```python
from build123d import *

# Parameters (mm, degrees)
SKETCH_1_R               = 75
EXTRUDE_1_DEPTH          = 20
F_4_0MM_1_D              = 4
PATTERN_CIRCULAR_1_COUNT = 4
PATTERN_CIRCULAR_2_COUNT = 6
CUT_EXTRUDE_1_REACH      = 109.935
SKETCH_7_R               = 5
F_4_0MM_2_D              = 4
PATTERN_CIRCULAR_3_COUNT = 2


with BuildPart() as part:
    # 草圖1 → 填料-伸長1 (new body)
    with BuildSketch(Plane.XY):
        Circle(SKETCH_1_R)
    extrude(amount=EXTRUDE_1_DEPTH)

    # Ø4.0mm 定位孔1 (through all)
    with Locations(Plane.XY.offset(20)):
        with Locations((29.69848481, 29.69848481)):
            f_4_0mm_1 = Hole(F_4_0MM_1_D / 2)

    # 環狀複製排列1: Ø4.0mm 定位孔1 ×4 about axis
    pattern_circular_1_axis = Axis((0, 0, 0), (0, 0, 1))
    for i in range(1, PATTERN_CIRCULAR_1_COUNT):
        add(f_4_0mm_1.rotate(pattern_circular_1_axis, i * 360 / PATTERN_CIRCULAR_1_COUNT), mode=Mode.SUBTRACT)

    # 草圖6 → Ø6.0mm 定位孔1 (revolve, cut)
    with BuildSketch(Plane(origin=(0, 75, 10), x_dir=(0, 0, 1), z_dir=(1, 0, 0))):
        Polygon((0, 0), (0, 21.802581857), (3, 20), (3, 0), align=None)
    f_6_0mm_1 = revolve(axis=Axis((0, 81.35, 10), (0, -1, 0)), mode=Mode.SUBTRACT)

    # 環狀複製排列2: Ø6.0mm 定位孔1 ×6 about axis
    pattern_circular_2_axis = Axis((0, 0, -88.99), (0, 0, 1))
    for i in range(1, PATTERN_CIRCULAR_2_COUNT):
        add(f_6_0mm_1.rotate(pattern_circular_2_axis, i * 360 / PATTERN_CIRCULAR_2_COUNT), mode=Mode.SUBTRACT)

    # 草圖7 → 除料-伸長1 (cut, up to next)
    with BuildSketch(Plane.XY.offset(20), mode=Mode.PRIVATE) as cut_extrude_1_sk1:
        Circle(SKETCH_7_R)
    cut_extrude_1_tool1 = extrude(cut_extrude_1_sk1.sketch, amount=-CUT_EXTRUDE_1_REACH, mode=Mode.PRIVATE) & part.part
    add(cut_extrude_1_tool1.solids().sort_by_distance((0, 0, 20))[0], mode=Mode.SUBTRACT)

    # Ø4.0mm 定位孔2 (through all)
    with Locations(Plane.XY.offset(20)):
        with Locations((-42, 0)):
            f_4_0mm_2 = Hole(F_4_0MM_2_D / 2)

    # 環狀複製排列3: Ø4.0mm 定位孔2 ×2 about axis
    pattern_circular_3_axis = Axis((0, 0, 0), (0, 0, 1))
    for i in range(1, PATTERN_CIRCULAR_3_COUNT):
        add(f_4_0mm_2.rotate(pattern_circular_3_axis, i * 360 / PATTERN_CIRCULAR_3_COUNT), mode=Mode.SUBTRACT)


solid = part.part
```
The listing builds one solid part. Answer for the finished solid, in the listing's coordinates (mm). A direction names the side the tool comes from. Give positions to 0.01 mm unless a question says otherwise; leave off trailing zeros. Order: outer loops, then holes, each group sorted by start corner. A loop starts at its lowest first (then second) coordinate and runs counter-clockwise, first axis right, second up.
Item 1: The part is cut by section C-C, the plane z = 15. Give the vertices of the cut face in (x, y).
From the geometry:
outline: circle Ø150 at (0, 0); hole circle Ø4 at (-42, 0); hole circle Ø4 at (-29.7, -29.7); hole circle Ø4 at (-29.7, 29.7); hole circle Ø10 at (0, 0); hole circle Ø4 at (29.7, -29.7); hole circle Ø4 at (29.7, 29.7); hole circle Ø4 at (42, 0)
Item 2: The part is cut by section A-A, the plane y = 0. Give the vertices of the cut face in (x, z).
From the geometry:
outline: (-75, 0) - (-44, 0) - (-44, 20) - (-75, 20) - close; (-40, 0) - (-5, 0) - (-5, 20) - (-40, 20) - close; (5, 0) - (40, 0) - (40, 20) - (5, 20) - close; (44, 0) - (75, 0) - (75, 20) - (44, 20) - close
Item 3: The part is cut by section D-D, the plane x = -15.5. Give the vertices of the cut face in (y, z).
From the geometry:
outline: (-73.38, 0) - (73.38, 0) - (73.38, 20) - (-73.38, 20) - close
Item 4: Find the intervals of material crossed by probe 1 along X at (y, z) = (30, 4.5); probe 2 along Y at (x, z) = (60.5, 7.75); probe 3 along X at (y, z) = (-28.5, 19), in increasing order.
From the geometry:
probe 1: x = -68.74 to -31.68, -27.72 to 27.72, 31.68 to 68.74
probe 2: y = -44.33 to -37.22, -32.64 to 32.64, 37.22 to 44.33
probe 3: x = -69.37 to -31.3, -28.1 to 28.1, 31.3 to 69.37
Item 5: The part is cut by section B-B, the plane x = 42. Give the vertices of the cut face in (y, z), and give its area (3 significant figures).
From the geometry:
outline: (-62.14, 0) - (-2, 0) - (-2, 20) - (-62.14, 20) - close; (2, 0) - (62.14, 0) - (62.14, 20) - (2, 20) - close
area: 2,410 mm2
Item 6: For a pull along Y with two mould halves and no side action, classify faces 4 (the face through (-31.3, -28.5, 9.9)), 5 (the face through (16, 1, 20)), 6 (the face through (0.2, 53.51, 10.48)) as pulls with the +Y half, pulls with the -Y half, needs draft (parallel to the pull), parting line crosses it, or undercut.
From the geometry:
face 4: undercut
face 5: needs draft
face 6: pulls with the +Y half
Item 7: Given pin 1 Ø1 at (y, z) = (12, 9.5) entering from -X; pin 2 Ø2 at (x, z) = (-57, 2) entering from +Y; pin 3 Ø3 at (x, z) = (40, 15.5) entering from +Y; pin 4 Ø2.5 at (x, y) = (29.7, 29.7) entering from +Z, each flat-ended and moving along its own axis, determine where each tip first touches the part or whether it passes through.
From the geometry:
pin 1: stops at x = -74.11
pin 2: stops at y = 49.89
pin 3: stops at y = 64.36
pin 4: passes through
Item 8: Which of the six approach directions +Z, -Z, +X, -X, +Y, -Y give full straight-line access (tool end or side, diameter ignored) to faces 1 (the face through (1.15, 65.14, 12.77)), 2 (the face through (27.85, 28.93, 9.86)), 3 (the face through (-46.561, 26.375, 10.28))?
From the geometry:
face 1: +Y
face 2: +Z, -Z
face 3: none
